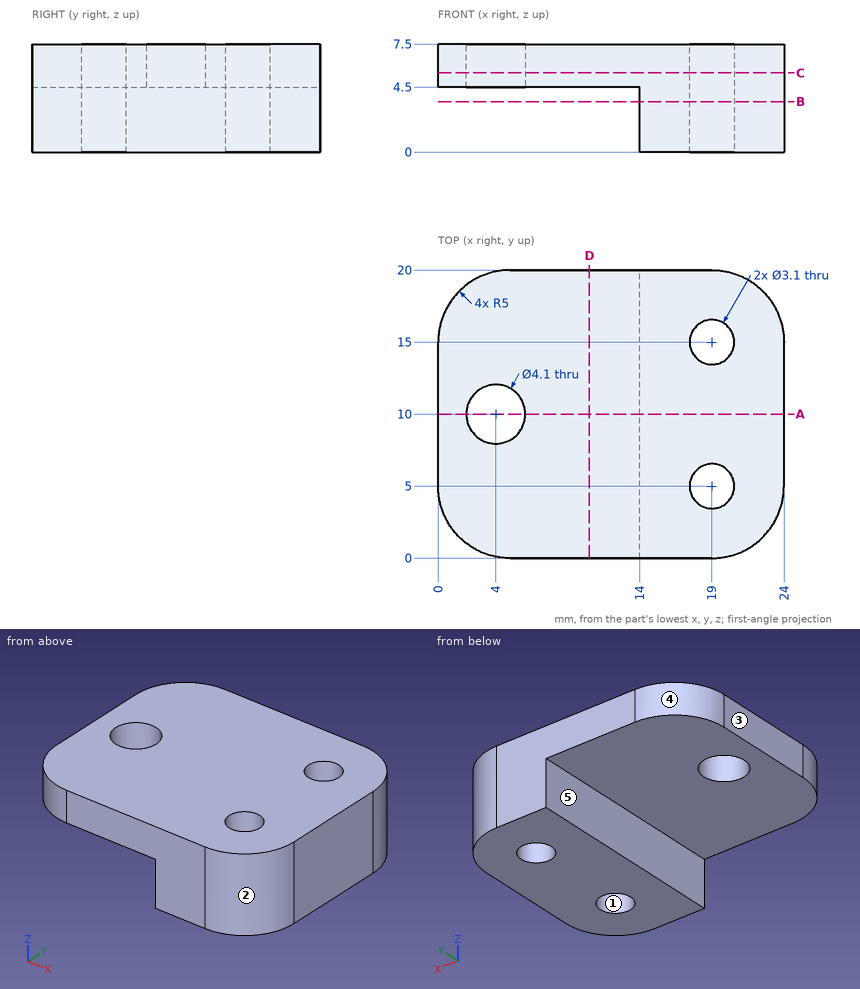
Here's the drawing with two shaded views (mm, measured from the low corner). I have some questions. A direction names the side the tool comes from. Coordinates: 2 decimals unless noted, no trailing zeros. Order: outer loops, then holes, each group sorted by start corner. A loop starts at its lowest first (then second) coordinate and runs counter-clockwise, first axis right, second up. Notation, with made-up numbers: (48, 26.25) - (99, 26.25) arc R13 ccw to (99, 35.25) - close; hole circle Ø1 at (-6, 85.5). An arc over 180 degrees is marked (long way). Answer in a Markdown table with one row per item. Add a question column.
(1) Will this pin go through, and if not, where does the flat tip stop? pin 1 (1.5 mm diameter, centred on x = 21, z = 6.5, fed in from +Y).
(2) If we mould it in two halves opening along Y, with no side actions, what happens to the marked faces 1, 2 and 3? For each: released by +Y, released by -Y, zero draft, split by the parting line, or undercut.
(3) I need wall thicknesses on L1, parallel to Y at x = 19, z = 2; L2, parallel to Z at x = 3.5, y = 14; L3, parallel to X at y = 7, z = 2.5. Which ranges of each line are inside material? Lowest first, please.
(4) If we section it at A-A, the plane y = 10: Please give me the cut outline in (x, z), then the cut area to 3 significant figures.
(5) If we section it at B-B, the plane z = 3.5: Please give me the cut outline in (x, y).
(6) If we section it at C-C, the plane z = 5.5: Please give me the cut outline in (x, y), then the cut area to 3 significant figures.
(7) On a 3-axis mill with a long thin cutter (end or side, diameter ignored), from which of +Z, -Z, +X, -X, +Y, -Y can I reach the whole of each face in a straight line? I mean the marked faces 4 and 5. Say none if no direction works.
(8) If we section it at D-D, the plane x = 10.5: Please give me the cut outline in (y, z), then the cut area to 3 significant figures.
Results are:
| question | item | result |
|---|---|---|
| 1 | pin 1 | stops at y = 19.84 |
| 2 | face 1 | undercut |
| 2 | face 2 | released by -Y |
| 2 | face 3 | zero draft |
| 3 | L1 | y = 0 to 3.45, 6.55 to 13.45, 16.55 to 20 |
| 3 | L2 | z = 4.5 to 7.5 |
| 3 | L3 | x = 14 to 24 |
| 4 | outline | (0, 4.5) - (1.95, 4.5) - (1.95, 7.5) - (0, 7.5) - close; (6.05, 4.5) - (14, 4.5) - (14, 0) - (24, 0) - (24, 7.5) - (6.05, 7.5) - close |
| 4 | area | 105 mm2 |
| 5 | outline | (14, 0) - (19, 0) arc R5 ccw to (24, 5) - (24, 15) arc R5 ccw to (19, 20) - (14, 20) - close; hole circle Ø3.1 at (19, 5); hole circle Ø3.1 at (19, 15) |
| 6 | outline | (0, 5) arc R5 ccw to (5, 0) - (19, 0) arc R5 ccw to (24, 5) - (24, 15) arc R5 ccw to (19, 20) - (5, 20) arc R5 ccw to (0, 15) - close; hole circle Ø4.1 at (4, 10); hole circle Ø3.1 at (19, 5); hole circle Ø3.1 at (19, 15) |
| 6 | area | 430 mm2 |
| 7 | face 4 | +Z, -Z, -X, +Y |
| 7 | face 5 | -Z, -X, +Y, -Y |
| 8 | outline | (0, 4.5) - (20, 4.5) - (20, 7.5) - (0, 7.5) - close |
| 8 | area | 60.0 mm2 |
